Job drawing, mm, ordinate dimensions from the low corner. One solid piece. Round coordinates to 2 decimals unless told otherwise and drop trailing zeros. Loops run counter-clockwise (first coordinate to the right, second up) from the corner with the lowest first, then second, coordinate; pieces in that order, holes last.
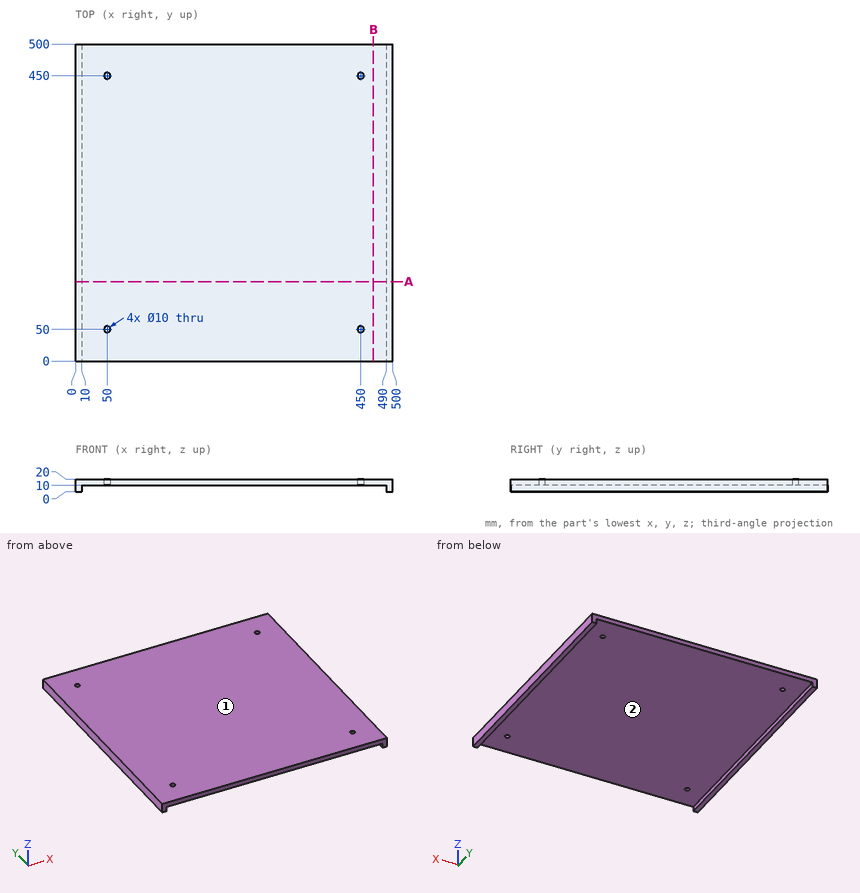
(1) Pull direction X, two halves, no side cores. Call the marked faces 1 and 2: +X half, -X half, draft (parallel to the pull), parting line (faces both ways), or undercut.
Responses:
face 1: draft
face 2: undercut
(2) Slice it at B-B on x = 470. List the corners of the cut face in (y, z).
Responses:
outline: (0, 10) - (500, 10) - (500, 20) - (0, 20) - close
(3) Probe line 1 (Y direction, x = 450, z = 13.75); line 2 (X direction, y = 96.5, z = 9). List the from-to ranges inside material, lowest first.
Responses:
line 1: y = 0 to 45, 55 to 445, 455 to 500
line 2: x = 0 to 10, 490 to 500
(4) Pin check, flat tips, straight feed: P1, Ø11.5, axis at x = 50, y = 50, coming from the +Z side; P2, Ø6, axis at x = 50, y = 450, coming from the -Z side; P3, Ø16, axis at x = 450, y = 450, coming from the -Z side. Stop position of each tip, or through.
Responses:
P1: stops at z = 20
P2: passes through
P3: stops at z = 10
(5) Slice it at A-A on y = 125. List the corners of the cut face in (x, z).
Responses:
outline: (0, 0) - (10, 0) - (10, 10) - (490, 10) - (490, 0) - (500, 0) - (500, 20) - (0, 20) - close
